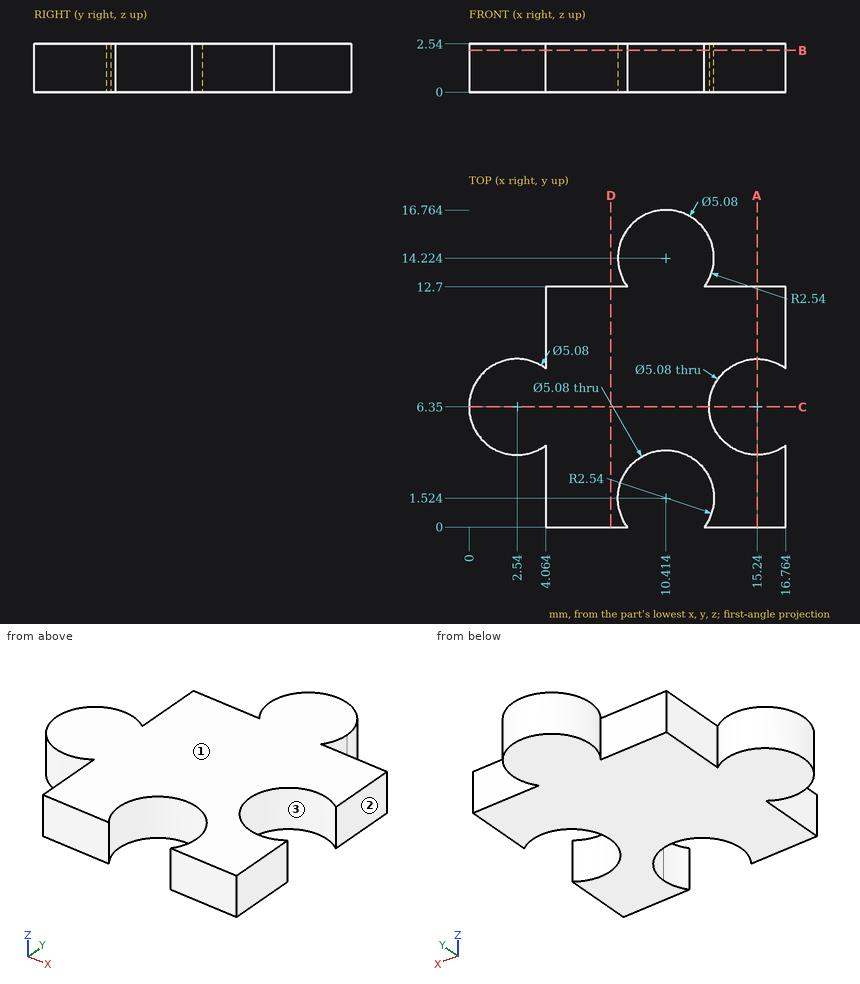
Source: three-view drawing plus pictorial views. Frame: mm from the lowest corner of the part. Give positions to 0.01 mm unless a question says otherwise; leave off trailing zeros. Order: outer loops, then holes, each group sorted by start corner. A loop starts at its lowest first (then second) coordinate and runs counter-clockwise, first axis right, second up. Notation, with made-up numbers: (73.5, 10) - (79.5, 10) arc R9 ccw to (79.5, 22) - close; hole circle Ø1 at (49, 3.25). An arc over 180 degrees is marked (long way). Answer as a JSON object with one key per item and string values. Group by question number.
Q1. First-contact query: pin 1 Ø1.3 at (y, z) = (11.5, 1.5) entering from -X. Flat tip, straight axial feed; report the tip coordinate or a pass-through.
Q2. Cut plane A-A, the plane x = 15.24. Output: boundary loops of the cut face in (y, z), then the cut area to 3 significant figures.
Q3. Cut plane C-C, the plane y = 6.35. Output: boundary loops of the cut face in (x, z), then the cut area to 3 significant figures.
Q4. Cut plane B-B, the plane z = 2.2. Output: boundary loops of the cut face in (x, y).
Q5. Line query: probe 1 along X at (y, z) = (1.5, 1.05); probe 2 along Y at (x, z) = (15.24, 1.7); probe 3 along X at (y, z) = (8.5, 1.25). Output: solid intervals per line, ascending.
Q6. Mould query, pull axis X, two halves, no side actions, for the marked faces 1, 2 and 3. Classes: pulls with the +X half, pulls with the -X half, needs draft (parallel to the pull), parting line crosses it, or undercut.
Results:
{
 "1": {"pin 1": "x = 4.06"},
 "2": {"outline": "(0, 0) - (3.81, 0) - (3.81, 2.54) - (0, 2.54) - close; (8.89, 0) - (12.7, 0) - (12.7, 2.54) - (8.89, 2.54) - close", "area": "19.4 mm^2"},
 "3": {"outline": "(0, 0) - (12.7, 0) - (12.7, 2.54) - (0, 2.54) - close", "area": "32.3 mm^2"},
 "4": {"outline": "(4.06, 0) - (8.38, 0) arc R2.54 cw (long way) to (12.45, 0) - (16.76, 0) - (16.76, 4.32) arc R2.54 cw (long way) to (16.76, 8.38) - (16.76, 12.7) - (12.45, 12.7) arc R2.54 ccw (long way) to (8.38, 12.7) - (4.06, 12.7) - (4.06, 8.38) arc R2.54 ccw (long way) to (4.06, 4.32) - close"},
 "5": {"probe 1": "4.06 to 7.87, 12.95 to 16.76", "probe 2": "0 to 3.81, 8.89 to 12.7", "probe 3": "1.19 to 3.89, 4.06 to 13.89, 16.59 to 16.76"},
 "6": {"face 1": "needs draft", "face 2": "pulls with the +X half", "face 3": "undercut"}
}
